from build123d import *

# Parameters (mm, degrees)
PAD019_DEPTH    = 200
SKETCH043_R     = 1.2
POCKET023_DEPTH = 15


with BuildPart() as body010:
    # Sketch042 → Pad019 (new body)
    with BuildSketch(Plane.XY):
        Polygon((0, 22), (15, 22), (15, 14.5), (14, 14.5), (14, 7.5), (15, 7.5), (15, 6.5), (14, 6.5), (14, 1.5), (15, 1.5), (15, 0), (0, 0), align=None)
    extrude(amount=PAD019_DEPTH)

    # Sketch043 (on Face7 of Pad019) → Pocket023 (cut)
    with BuildSketch(Plane(origin=(0, 0, 0), x_dir=(0, -1, 0), z_dir=(-1, 0, 0))):
        with Locations((-11, 5)):
            Circle(SKETCH043_R)
        with Locations((-11, 35)):
            Circle(SKETCH043_R)
        with Locations((-11, 65)):
            Circle(SKETCH043_R)
        with Locations((-11, 110)):
            Circle(SKETCH043_R)
        with Locations((-11, 95)):
            Circle(SKETCH043_R)
        with Locations((-11, 80)):
            Circle(SKETCH043_R)
        with Locations((-11, 50)):
            Circle(SKETCH043_R)
        with Locations((-11, 20)):
            Circle(SKETCH043_R)
        with Locations((-11, 140)):
            Circle(SKETCH043_R)
        with Locations((-11, 125)):
            Circle(SKETCH043_R)
        with Locations((-11, 155)):
            Circle(SKETCH043_R)
    extrude(amount=-POCKET023_DEPTH, mode=Mode.SUBTRACT)


with BuildPart() as body010_1:
    # Body010 placement: moved
    add(body010.part.moved(Location((-123, 78, -111))))


with BuildPart() as part_mirroring001:
    # Part__Mirroring001: instance of Body010
    add(body010_1.part.mirror(Plane(origin=(0, 0, 0), x_dir=(0, -1, 0), z_dir=(1, 0, 0))))


solid = part_mirroring001.part
Geometry: final body of the model. Coordinates: model frame, mm. A direction names the side the tool comes from. Coordinates: 2 decimals unless noted, no trailing zeros. Write each loop counter-clockwise with the first axis right and the second up, starting at its lowest first coordinate (ties: lowest second). Pieces come first, ordered by that corner, then holes. Notation, with made-up numbers: (56, -26.75) - (103, -26.75) arc R21 ccw to (103, -8.75) - close; hole circle Ø10 at (89, 66). An arc over 180 degrees is marked (long way). Return JSON: item names as keys, results as strings.
Item 1: Line query: L1, parallel to Y at x = 108.5, z = 44; L2, parallel to Y at x = 113.25, z = 29; L3, parallel to X at y = 89.25, z = -92.5. Output: solid intervals per line, ascending.
Completed:
{"L1": "y = 78 to 79.5, 84.5 to 85.5, 92.5 to 100", "L2": "y = 78 to 87.8, 90.2 to 100", "L3": "x = 109 to 123"}
Item 2: Reachability of faces 4 (the face through (115, 89, -111)), 5 (the face through (109, 89, -12)) from +Z, -Z, +X, -X, +Y, -Y: full face, straight path, thin tool, end or side. Return the list, or none.
Completed:
{"face 4": "-Z, +X, -X, +Y, -Y", "face 5": "+Z, -Z, -X"}
Item 3: Pin query (flat end, axial travel): pin 1 Ø3 at (y, z) = (89, -46) entering from -X; pin 2 Ø2 at (y, z) = (89, -91) entering from -X. Return the tip coordinate at first contact, or that it passes through.
Completed:
{"pin 1": "stops at x = 109", "pin 2": "passes through"}
Item 4: Pull-direction query (Y, two-part tool) for faces 1 (the face through (115, 78, -12)), 2 (the face through (109, 82, -12)), 3 (the face through (108, 96, -12)); classes: +Y half, -Y half, draft (parallel to the pull), parting line (faces both ways), or undercut.
Completed:
{"face 1": "-Y half", "face 2": "undercut", "face 3": "draft"}
Item 5: Section query A-A (z = 32). Output: boundary loops of the cut face in (x, y), and give its area (3 significant figures).
Completed:
{"outline": "(108, 78) - (123, 78) - (123, 100) - (108, 100) - (108, 92.5) - (109, 92.5) - (109, 85.5) - (108, 85.5) - (108, 84.5) - (109, 84.5) - (109, 79.5) - (108, 79.5) - close", "area": "318 mm2"}
